Build history of the part. All positions in model axes, mm. A direction names the side the tool comes from. Give positions to 0.01 mm unless a question says otherwise; leave off trailing zeros. Write each loop counter-clockwise with the first axis right and the second up, starting at its lowest first coordinate (ties: lowest second). Pieces come first, ordered by that corner, then holes. Notation, with made-up numbers: M 27,-29.5 L 82,-29.5 A22 cw 82,-18.5 Z; hole C -4,-31.75 d2. An arc over 180 degrees is marked long. One line per item, written item: value. Start each with the question number.
from build123d import *

# Parameters (mm, degrees)
SKETCH1_R               = 11
BOSS_EXTRUDE1_DEPTH     = 3.5
CUT_EXTRUDE1_DEPTH      = 16.945218719
CUT_EXTRUDE1_DEPTH_BACK = 16.945218719
SKETCH2_R               = 10
SKETCH3_R               = 10
BOSS_EXTRUDE2_DEPTH     = 2.75
CUT_EXTRUDE2_DEPTH      = 16.945218719
CUT_EXTRUDE2_DEPTH_BACK = 16.945218719
SKETCH4_R               = 4.75
SKETCH5_R               = 4.75
BOSS_EXTRUDE3_DEPTH     = 3.5
CUT_EXTRUDE3_DEPTH      = 16.945218719
CUT_EXTRUDE3_DEPTH_BACK = 16.945218719
SKETCH6_R               = 4.05
FILLET1_R               = 0.5


with BuildPart() as part:
    # Sketch1 → Boss-Extrude1 (new, symmetric)
    with BuildSketch(Plane(origin=(0, 0, 0), x_dir=(1, 0, 0), z_dir=(0, 1, 0))):
        with Locations(Location((0, 0, 0), (0, 0, 270))):
            Circle(SKETCH1_R)
    extrude(amount=BOSS_EXTRUDE1_DEPTH, both=True)

    # Sketch2 → Cut-Extrude1 (cut, two sides: drawn at the far end of the back side and taken through both)
    with BuildSketch(Plane(origin=(0, 0, 0), x_dir=(1, 0, 0), z_dir=(0, 1, 0)).offset(-CUT_EXTRUDE1_DEPTH_BACK)):
        with Locations(Location((0, 0, 0), (0, 0, 270))):
            Circle(SKETCH2_R)
    extrude(amount=CUT_EXTRUDE1_DEPTH + CUT_EXTRUDE1_DEPTH_BACK, mode=Mode.SUBTRACT)

    # Sketch3 → Boss-Extrude2 (add, symmetric)
    with BuildSketch(Plane(origin=(0, 0, 0), x_dir=(1, 0, 0), z_dir=(0, 1, 0))):
        with Locations(Location((0, 0, 0), (0, 0, 270))):
            Circle(SKETCH3_R)
    extrude(amount=BOSS_EXTRUDE2_DEPTH, both=True)

    # Sketch4 → Cut-Extrude2 (cut, two sides: drawn at the far end of the back side and taken through both)
    with BuildSketch(Plane(origin=(0, 0, 0), x_dir=(1, 0, 0), z_dir=(0, 1, 0)).offset(-CUT_EXTRUDE2_DEPTH_BACK)):
        with Locations(Location((0, 0, 0), (0, 0, 270))):
            Circle(SKETCH4_R)
    extrude(amount=CUT_EXTRUDE2_DEPTH + CUT_EXTRUDE2_DEPTH_BACK, mode=Mode.SUBTRACT)

    # Sketch5 → Boss-Extrude3 (add, symmetric)
    with BuildSketch(Plane(origin=(0, 0, 0), x_dir=(1, 0, 0), z_dir=(0, 1, 0))):
        with Locations(Location((0, 0, 0), (0, 0, 270))):
            Circle(SKETCH5_R)
    extrude(amount=BOSS_EXTRUDE3_DEPTH, both=True)

    # Sketch6 → Cut-Extrude3 (cut, two sides: drawn at the far end of the back side and taken through both)
    with BuildSketch(Plane(origin=(0, 0, 0), x_dir=(1, 0, 0), z_dir=(0, 1, 0)).offset(-CUT_EXTRUDE3_DEPTH_BACK)):
        with Locations(Location((0, 0, 0), (0, 0, 270))):
            Circle(SKETCH6_R)
    extrude(amount=CUT_EXTRUDE3_DEPTH + CUT_EXTRUDE3_DEPTH_BACK, mode=Mode.SUBTRACT)

    # Fillet1
    fillet1_edges = [part.edges().sort_by_distance(p)[0] for p in [
        (0, -3.5, -11),
        (0, 3.5, -11),
        (0, -3.5, -10),
        (0, 3.5, -10),
    ]]
    fillet(fillet1_edges, radius=FILLET1_R - 0.0001)  # a hair under: the kernel refuses the full size


solid = part.part
1) Probe line 1 along X through (y, z) = (2.9, 0); line 2 along X through (y, z) = (-2, 0); line 3 along Y through (x, z) = (2.5, 8.75). List the from-to ranges inside material, lowest first. Write a range as from..to.
2) Tool access for faces 1 (the face through (-2.89, -3.12, -3.77)), 2 (the face through (-2.89, 3.13, -3.77)), 3 (the face through (4, 3.5, -2)): list every direction of +Z, -Z, +X, -X, +Y, -Y with a clear straight run to the whole face (end or side of a thin tool).
3) Drop flat-ended pins along their axis: P1, Ø1.5, axis at x = 3, y = 0.5, coming from the -Z side; P2, Ø5, axis at x = 0, z = 0, coming from the +Y side; P3, Ø1.5, axis at x = -7, z = 6, coming from the -Y side; P4, Ø1.5, axis at x = -5, y = 0, coming from the +Z side. Give the stop position or say it passes through.
4) Mould opens along Z. For faces 4 (the face through (4, -3.5, -2)), 5 (the face through (2.4, -2.75, 4.3)), 6 (the face through (-10.74, 0.04, -2.38)) say: released by +Z, released by -Z, zero draft, split by the parting line, or undercut.
5) Band-saw the part on C-C (y = -1). List the corners of the cut face in (x, z), then the cut area to 3 significant figures.
Model answer:
1. line 1: x = -11..-10, -4.75..-4.05, 4.05..4.75, 10..11
1. line 2: x = -11..-4.05, 4.05..11
1. line 3: y = -2.75..2.75
2. face 1: -Y
2. face 2: +Y
2. face 3: +Z, -Z, +X, -X, +Y
3. P1: stops at z = -10.77
3. P2: passes through
3. P3: stops at y = -2.75
3. P4: stops at z = 10.15
4. face 4: zero draft
4. face 5: undercut
4. face 6: split by the parting line
5. outline: C 0,0 d22; hole C 0,0 d8.1
5. area: 329 mm²
